from build123d import *

# Parameters (mm, degrees)
SKETCH_2_W                       = 1.5
SKETCH_2_H                       = 231.5
SM_BASE_FLANGE_1_DEPTH           = 265
SKETCH_3_W                       = 2.488275725
SKETCH_3_H                       = 14
CUT_EXTRUDE_1_DEPTH              = 8
SKETCH_4_W                       = 80
SKETCH_4_H                       = 10
CUT_EXTRUDE_2_DEPTH              = 6
SM_EDGE_FLANGE_1_STRIP_W         = 7.4732
SM_EDGE_FLANGE_1_STRIP_H         = 1.5
SM_EDGE_FLANGE_1_STRIP_CUT_DEPTH = 265
SM_EDGE_FLANGE_1_DEPTH           = 265
SKETCH_10_W                      = 163
SKETCH_10_H                      = 1.5
EXTRUDE_1_DEPTH                  = 130.17
SKETCH_11_W                      = 38.16564302
SKETCH_11_H                      = 1.5
EXTRUDE_2_DEPTH                  = 130.17
SKETCH_12_R                      = 2.75
CUT_EXTRUDE_3_DEPTH              = 20
SKETCH_13_R                      = 2.75
CUT_EXTRUDE_4_DEPTH              = 10
SKETCH_14_W                      = 13.490100929
SKETCH_14_H                      = 1.5
CUT_EXTRUDE_5_DEPTH              = 2
SKETCH_15_R                      = 2.25
CUT_EXTRUDE_6_DEPTH              = 10


# Sheet-metal steps are written as plain solids
with BuildPart() as part:
    # Sketch 2 → 基体-法兰1 (new body)
    with BuildSketch(Plane.XY):
        with Locations((0.75, 115.75)):
            Rectangle(SKETCH_2_W, SKETCH_2_H)
    extrude(amount=SM_BASE_FLANGE_1_DEPTH)

    # 草图3 → 切除-拉伸1 (cut)
    with BuildSketch(Plane(origin=(0, 231.5, 0), x_dir=(1, 0, 0), z_dir=(0, 1, 0))):
        with Locations((1.244137863, -258)):
            Rectangle(SKETCH_3_W, SKETCH_3_H)
    extrude(amount=-CUT_EXTRUDE_1_DEPTH, mode=Mode.SUBTRACT)

    # 草图4 → 切除-拉伸2 (cut)
    with BuildSketch(Plane.ZY):
        with Locations((192.56107144, 61.95061584)):
            Rectangle(SKETCH_4_W, SKETCH_4_H)
    extrude(amount=-CUT_EXTRUDE_2_DEPTH, mode=Mode.SUBTRACT)

    # 边线-法兰1 strip (across the edge) → 边线-法兰1 strip cut (cut)
    with BuildSketch(Plane(origin=(0, 0, 0), x_dir=(0, 1, 0), z_dir=(0, 0, 1))):
        with Locations((-1.5, -0.75)):
            Rectangle(SM_EDGE_FLANGE_1_STRIP_W, SM_EDGE_FLANGE_1_STRIP_H)
    extrude(amount=SM_EDGE_FLANGE_1_STRIP_CUT_DEPTH, mode=Mode.SUBTRACT)

    # 边线-法兰1 section (across the edge) → 边线-法兰1 (add)
    with BuildSketch(Plane(origin=(0, 0, 0), x_dir=(0, 1, 0), z_dir=(0, 0, 1))):
        with BuildLine():
            Line((0, 0.7366), (0, 318.5))
            Line((0, 318.5), (1.5, 318.5))
            Line((1.5, 318.5), (1.5, 0.7366))
            ThreePointArc((1.5, 0.7366), (1.715745145, 0.215745145), (2.2366, 0))
            Line((2.2366, 0), (2.2366, -1.5))
            ThreePointArc((2.2366, -1.5), (0.655084973, -0.844915027), (0, 0.7366))
        make_face()
    extrude(amount=SM_EDGE_FLANGE_1_DEPTH)

    # 草图10 → 凸台-拉伸1 (add)
    with BuildSketch(Plane.ZY.offset(318.5)):
        with Locations((81.5, 0.75)):
            Rectangle(SKETCH_10_W, SKETCH_10_H)
    extrude(amount=EXTRUDE_1_DEPTH)

    # 草图11 → 凸台-拉伸2 (add)
    with BuildSketch(Plane.ZY.offset(318.5)):
        with Locations((245.91717849, 0.75)):
            Rectangle(SKETCH_11_W, SKETCH_11_H)
    extrude(amount=EXTRUDE_2_DEPTH)

    # 草图12 → 切除-拉伸3 (cut)
    with BuildSketch(Plane(origin=(1.5, 0, 0), x_dir=(0, 0, -1), z_dir=(1, 0, 0))):
        with Locations((-258.6183, 162.5)):
            Circle(SKETCH_12_R)
        with Locations((-258.6183, 112.5)):
            Circle(SKETCH_12_R)
        with Locations((-258.6183, 62.5)):
            Circle(SKETCH_12_R)
    extrude(amount=-CUT_EXTRUDE_3_DEPTH, mode=Mode.SUBTRACT)

    # 草图13 → 切除-拉伸4 (cut)
    with BuildSketch(Plane.XZ):
        with Locations((-352.4684, 258.6183)):
            Circle(SKETCH_13_R)
        with Locations((-232.4684, 258.6183)):
            Circle(SKETCH_13_R)
        with Locations((-112.4684, 258.6183)):
            Circle(SKETCH_13_R)
    extrude(amount=-CUT_EXTRUDE_4_DEPTH, mode=Mode.SUBTRACT)

    # 草图14 → 切除-拉伸5 (cut)
    with BuildSketch(Plane.ZY.offset(448.67)):
        with Locations((258.254949536, 0.75)):
            Rectangle(SKETCH_14_W, SKETCH_14_H)
    extrude(amount=-CUT_EXTRUDE_5_DEPTH, mode=Mode.SUBTRACT)

    # 草图15 → 切除-拉伸6 (cut)
    with BuildSketch(Plane(origin=(1.5, 0, 0), x_dir=(0, 0, -1), z_dir=(1, 0, 0))):
        with Locations((-45.5, 228.5)):
            Circle(SKETCH_15_R)
        with Locations((-85.5, 228.5)):
            Circle(SKETCH_15_R)
        with Locations(Location((-205.5, 228.5, 0), (0, 0, 180))):
            Circle(SKETCH_15_R)
        with Locations(Location((-165.5, 228.5, 0), (0, 0, 180))):
            Circle(SKETCH_15_R)
    extrude(amount=-CUT_EXTRUDE_6_DEPTH, mode=Mode.SUBTRACT)


solid = part.part
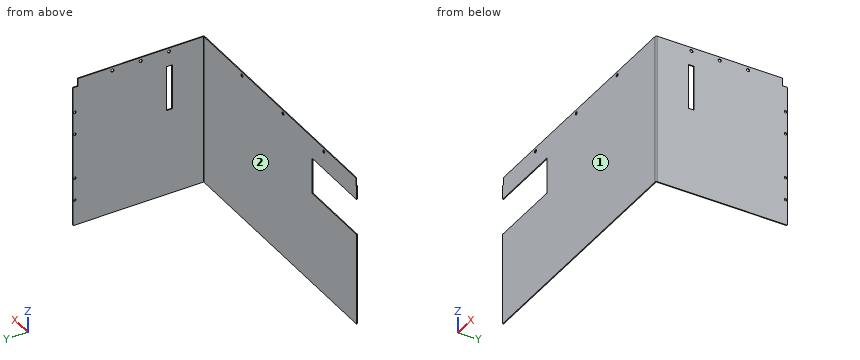
Design review of the part built by this model. Coordinates are the model's own, in mm. Face numbers are marked on the shaded views. A direction names the side the tool comes from. Give positions to 0.01 mm unless a question says otherwise; leave off trailing zeros. Order: outer loops, then holes, each group sorted by start corner. A loop starts at its lowest first (then second) coordinate and runs counter-clockwise, first axis right, second up. Notation, with made-up numbers: (-31, 25) - (19, 25) arc R29 ccw to (19, 58) - close; hole circle Ø4 at (65.5, 43.25). An arc over 180 degrees is marked (long way). Use CSV: the item, a comma, the result in double quotes. Start each with the question number.
Q1. Take a section at C-C (y = 152). State the section outline as (x, z) points, and give its area (4 significant figures).
Q2. Take a section at A-A (x = -327.5). State the section outline as (y, z) points.
Q3. Take a section at B-B (z = 58.5). State the section outline as (x, y) points.
Q4. Machinability: for the marked faces 1 and 2, which of the approach directions +Z, -Z, +X, -X, +Y, -Y give a long, thin tool a straight path to every point of the face, cutting with its end or side? Answer none if there is none.
Q5. For line 1 (X direction, y = 206.5, z = 254); line 2 (Y direction, x = 0.45, z = 205.5), list the stretches that pass through material, from the lowest coordinate up.
Q6. For P1, Ø1.6, axis at y = 0.5, z = 255.5, coming from the -X side; P2, Ø1.2, axis at x = 0.5, z = 260, coming from the +Y side; P3, Ø4.5, axis at y = 62.5, z = 258.62, coming from the -X side; P4, Ø0.8, axis at y = 0.5, z = 209, coming from the -X side, all flat-tipped, find the tip position at first contact; note any pin that passes through.
Calculated:
1,outline,"(0, 0) - (1.5, 0) - (1.5, 265) - (0, 265) - close"
1,area,"397.5 mm²"
2,outline,"(0, 0) - (1.5, 0) - (1.5, 163) - (0, 163) - close; (0, 226.83) - (1.5, 226.83) - (1.5, 265) - (0, 265) - close"
3,outline,"(-448.67, 0) - (-0.74, 0) arc R2.24 ccw to (1.5, 2.24) - (1.5, 231.5) - (0, 231.5) - (0, 2.24) arc R0.74 cw to (-0.74, 1.5) - (-448.67, 1.5) - close"
4,face 1,"+Z, -Z, +X, -X, -Y"
4,face 2,"+Z, -Z, -X, +Y"
5,line 1,"x = 0 to 1.5"
5,line 2,"y = 0.34 to 56.95, 66.95 to 226.25, 230.75 to 231.5"
6,P1,"stops at x = -446.67"
6,P2,"stops at y = 223.5"
6,P3,"passes through"
6,P4,"stops at x = -318.5"
